Could you check a few things on this model? Use its own coordinates, in mm. Face numbers are marked on the shaded views. A direction names the side the tool comes from. Give positions to 0.01 mm unless a question says otherwise; leave off trailing zeros. Order: outer loops, then holes, each group sorted by start corner. A loop starts at its lowest first (then second) coordinate and runs counter-clockwise, first axis right, second up. Notation, with made-up numbers: M -39.5,7.5 L -18.5,7.5 A31 ccw -18.5,38.5 Z; hole C -18,5 d11. An arc over 180 degrees is marked long. Answer in a Markdown table with one row per item. Add a question column.
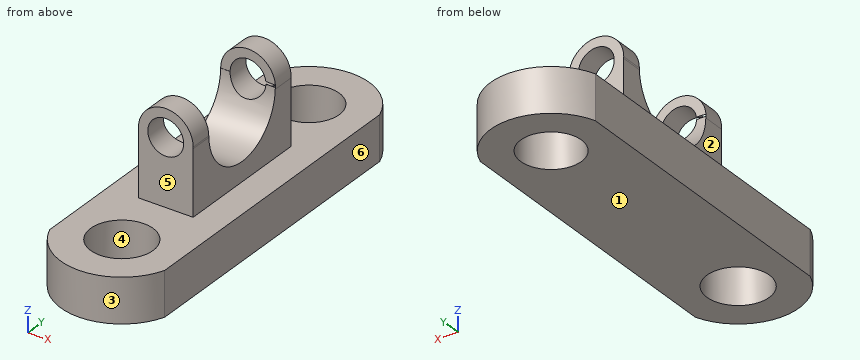
```python
from build123d import *

# Parameters (mm, degrees)
F0_R      = 17.8353013773
F0_R_2    = 17.3294738688
F1_DEPTH  = 25.4
F2_W      = 31.2288608402
F2_H      = 79.752035439
F3_DEPTH  = 38.1
F5_DEPTH  = 50.8
F7_DEPTH  = 12.7
F9_DEPTH  = 12.7
F10_R     = 10.2407588529
F11_DEPTH = 1270


with BuildPart() as f1:
    # F0 (on Top) → F1 (new body)
    with BuildSketch(Plane.XY):
        with BuildLine():
            Line((32.7898040414, -87.5596180558), (32.7898040414, 87.5596180558))
            ThreePointArc((32.7898040414, 87.5596180558), (0, 111.2754727593), (-32.7898040414, 87.5596180558))
            Line((-32.7898040414, 87.5596180558), (-32.7898040414, -87.5596180558))
            ThreePointArc((-32.7898040414, -87.5596180558), (0, -110.5480583126), (32.7898040414, -87.5596180558))
        make_face()
        with Locations((0, -75.6687968969)):
            Circle(F0_R, mode=Mode.SUBTRACT)
        with Locations((0, 76.7497718334)):
            Circle(F0_R_2, mode=Mode.SUBTRACT)
    extrude(amount=F1_DEPTH)

    # F2 (on face) → F3 (join)
    with BuildSketch(Plane.XY.offset(25.4)):
        Rectangle(F2_W, F2_H)
    extrude(amount=F3_DEPTH)

    # F4 (on face) → F5 (cut)
    with BuildSketch(Plane(origin=(-15.6144304201, 0, 0), x_dir=(0, -1, 0), z_dir=(-1, 0, 0))):
        with BuildLine():
            ThreePointArc((-27.0720647406, 63.5), (0, 36.4279352594), (27.0720647406, 63.5))
            Line((27.0720647406, 63.5), (-27.0720647406, 63.5))
        make_face()
    extrude(amount=-F5_DEPTH, mode=Mode.SUBTRACT)

    # F6 (on face) → F7 (join)
    with BuildSketch(Plane(origin=(0, 39.8760177195, 0), x_dir=(-1, 0, 0), z_dir=(0, 1, 0))):
        with BuildLine():
            ThreePointArc((15.6144304201, 62.5617992852), (15.6355493835, 63.0306883743), (15.6425911513, 63.5))
            ThreePointArc((15.6425911513, 63.5), (-0.4693116257, 79.1355493835), (-15.6144304201, 62.5617992852))
            Line((-15.6144304201, 62.5617992852), (-15.6144304201, 63.5))
            Line((-15.6144304201, 63.5), (15.6144304201, 63.5))
            Line((15.6144304201, 63.5), (15.6144304201, 62.5617992852))
        make_face()
    extrude(amount=-F7_DEPTH)

    # F8 (on face) → F9 (join)
    with BuildSketch(Plane.XZ.offset(39.8760177195)):
        with BuildLine():
            ThreePointArc((15.6144304201, 62.5804341006), (15.6347195512, 63.0400181066), (15.6414845455, 63.5))
            ThreePointArc((15.6414845455, 63.5), (-0.4599818934, 79.1347195512), (-15.6144304201, 62.5804341006))
            Line((-15.6144304201, 62.5804341006), (-15.6144304201, 63.5))
            Line((-15.6144304201, 63.5), (15.6144304201, 63.5))
            Line((15.6144304201, 63.5), (15.6144304201, 62.5804341006))
        make_face()
    extrude(amount=-F9_DEPTH)

    # F10 (on face) → F11 (cut)
    with BuildSketch(Plane.XZ.offset(39.8760177195)):
        with Locations((0, 63.5)):
            Circle(F10_R)
    extrude(amount=-F11_DEPTH, mode=Mode.SUBTRACT)


solid = f1.part
```
1. Suppose I cut it at D-D on y = 0. List the corners of the cut face in (x, z) for me, plus the area to 3 significant figures.
2. Will these pins go through, and if not, where does the flat tip stop? P1, Ø3, axis at x = 17, y = 61.5, coming from the +Z side; P2, Ø13, axis at x = 7, z = 67, coming from the +Y side; P3, Ø15.5, axis at x = -3.5, z = 62.5, coming from the -Y side; P4, Ø8, axis at y = -51.5, z = 27, coming from the +X side.
3. Suppose I cut it at C-C on z = 41. List the corners of the cut face in (x, y) for me.
4. Suppose I cut it at A-A on x = 0. List the corners of the cut face in (y, z) for me.
5. For the marked faces 5 and 6, which set-ups out of +Z, -Z, +X, -X, +Y, -Y let a thin tool reach every point of the face, with its end or its side?
6. Thinking about a two-plate mould opening in X: for the marked faces 1, 2, 3 and 4, which applies, pulls with the +X half, pulls with the -X half, needs draft (parallel to the pull), parting line crosses it, or undercut?
7. Suppose I cut it at B-B on y = -36.5. List the corners of the cut face in (x, z) for me.
8. If I drill on line 1 along Y through (x, z) = (0, 13); line 2 along Y through (x, z) = (-2, 18); line 3 along X through (y, z) = (-31, 63), over which ranges is the centre line in solid material (lowest first)? Write a range as [from, to].
Findings below:
| question | item | result |
|---|---|---|
| 1 | outline | M -32.79,0 L 32.79,0 L 32.79,25.4 L 15.61,25.4 L 15.61,36.43 L -15.61,36.43 L -15.61,25.4 L -32.79,25.4 Z |
| 1 | area | 2,010 mm2 |
| 2 | P1 | z = 25.4 |
| 2 | P2 | y = 39.88 |
| 2 | P3 | y = -39.88 |
| 2 | P4 | x = 32.79 |
| 3 | outline | M -15.61,-39.88 L 15.61,-39.88 L 15.61,-15.05 L -15.61,-15.05 Z; M -15.61,15.05 L 15.61,15.05 L 15.61,39.88 L -15.61,39.88 Z |
| 4 | outline | M -110.55,0 L -93.5,0 L -93.5,25.4 L -110.55,25.4 Z; M -57.83,0 L 59.42,0 L 59.42,25.4 L 39.88,25.4 L 39.88,53.26 L 25.06,53.26 A27.07 cw -25.06,53.26 L -39.88,53.26 L -39.88,25.4 L -57.83,25.4 Z; M -39.88,73.74 L -27.18,73.74 L -27.18,79.14 L -39.88,79.14 Z; M 27.18,73.74 L 39.88,73.74 L 39.88,79.14 L 27.18,79.14 Z; M 94.08,0 L 111.28,0 L 111.28,25.4 L 94.08,25.4 Z |
| 5 | face 5 | +Z, +X, -X, -Y |
| 5 | face 6 | +Z, -Z, +X, +Y, -Y |
| 6 | face 1 | needs draft |
| 6 | face 2 | pulls with the -X half |
| 6 | face 3 | parting line crosses it |
| 6 | face 4 | undercut |
| 7 | outline | M -32.79,0 L 32.79,0 L 32.79,25.4 L 15.61,25.4 L 15.61,62.58 A15.64 ccw long -15.61,62.58 L -15.61,25.4 L -32.79,25.4 Z; hole C 0,63.5 d20.48 |
| 8 | line 1 | [-110.55, -93.5], [-57.83, 59.42], [94.08, 111.28] |
| 8 | line 2 | [-110.49, -93.39], [-57.95, 59.54], [93.96, 111.22] |
| 8 | line 3 | [-15.63, -10.23], [10.23, 15.63] |
